Geometry check sheet. Reference: the model listing, model coordinates, mm. A direction names the side the tool comes from. Give positions to 0.01 mm unless a question says otherwise; leave off trailing zeros. Write each loop counter-clockwise with the first axis right and the second up, starting at its lowest first coordinate (ties: lowest second). Pieces come first, ordered by that corner, then holes.
(1) Thickness scan on line 1 along Z through (x, y) = (0.55, 0); line 2 along Y through (x, z) = (0.15, 3.25); line 3 along Y through (x, z) = (0.7, 2). Record the ranges inside material, lowest first.
(2) Tool access check on faces 4 (the flat face through (0.431, -1.248, 6.272)), 5 (the flat face through (0.431, 5.317, -3.553)), 6 (the flat face through (0.431, -6.272, -1.248)), 7 (the flat face through (0.431, 6.272, 1.248)). Record the directions out of +Z, -Z, +X, -X, +Y, -Y that give a thin tool (end or side, any length) a straight path to the whole face; none if there is none.
(3) Cross-section at A-A (y = 0). Record the boundary of the cut face in (x, z), and give its area (3 significant figures).
(4) Mould release check, pull along Y, two halves, no side actions. Record for faces 1 (the flat face through (0, -3.1, 3.1)), 2 (the cylindrical face through (0.43, -3.97, -3.95)), 3 (the flat face through (0.431, -3.553, 5.317)): +Y half, -Y half, draft (parallel to the pull), parting line (faces both ways), or undercut.
Autodesk Inventor part; units mm, degrees
ref_plane "Work Plane1" through (0, 0, 0) normal (0, -1, 0) x (1, 0, 0)
ref_plane "YZ Plane" through (0, 0, 0) normal (1, 0, 0) x (0, 1, 0)
ref_plane "XZ Plane" through (0, 0, 0) normal (0, 1, 0) x (-1, 0, 0)
sketch "Sketch1" plane through (0, 0, 0) normal (1, 0, 0) x (0, 1, 0)
  circle A0 centre (0, 0) radius 7
  circle A1 centre (0, 0) radius 4.2
  dimension "d0" = 14
  dimension "d1" = 8.4
extrude "Body" add sketch "Sketch1" along normal blind 0.85
sketch "Sketch2" plane through (0.85, 0, 0) normal (1, 0, 0) x (0, 0, -1)
  circle A0 centre (0, 0) radius 7
  line L0 (0, 0) -> (0, 7) construction
  arc A1 (1.3656, 6.8655) -> (-1.3656, 6.8655) centre (0, 0) ccw
  arc A2 (1.0925, 5.4924) -> (-1.0925, 5.4924) centre (0, 0) ccw
  line L1 (-1.0925, 5.4924) -> (-1.3656, 6.8655)
  line L2 (1.0925, 5.4924) -> (1.3656, 6.8655)
  line L3 (-1.0925, 5.4924) -> (0, 0) construction
  line L4 (0, 0) -> (1.0925, 5.4924) construction
  dimension "d4" = 22.5
  dimension "d5" = 11.2
extrude "Cut" cut sketch "Sketch2" against normal through all contours L2 A2 L1 A0 picked at (0.1221, 6.5193)
fillet "Fillet1" radius 0.21 2 edges at (0.425, 5.4924, 1.0925) (0.425, 5.4924, -1.0925)
pattern_circular "Cuts" count 8 over 360 about axis through (0, 0, 0) along (1, 0, 0) of "Cut", "Fillet1"
ref_plane "Work Plane1" through (0, 0, 0) normal (0, -1, 0) x (1, 0, 0)
equation "\"d0\" = SD2"
equation "\"d1\" = SD1"
equation "\"d2\" = SD"
equation "\"d5\" = 0.5 * SD2 + 0.5 * SD1"
equation "\"d6\" = SD"
equation "\"d8\" = 0.015 * SD2"
equation "\"SD\" = 0.85"
equation "\"SD1\" = 8.4"
equation "\"SD2\" = 14"
equation "\"NND\" = 8"
properties part number "AS 1969 - M8" material "Steel, Mild"
Reply:
1. line 1: z = -5.6 to -4.2, 4.2 to 5.6
1. line 2: y = -6.2 to -4.86, -4.56 to -2.66, 2.66 to 4.56, 4.86 to 6.2
1. line 3: y = -6.71 to -3.69, 3.69 to 6.71
2. face 4: +Z, +X, -X
2. face 5: -Z, +X, -X
2. face 6: +X, -X, -Y
2. face 7: +X, -X, +Y
3. outline: (0, -5.6) - (0.85, -5.6) - (0.85, -4.2) - (0, -4.2) - close; (0, 4.2) - (0.85, 4.2) - (0.85, 5.6) - (0, 5.6) - close
3. area: 2.38 mm2
4. face 1: draft
4. face 2: undercut
4. face 3: -Y half
